```python
from build123d import *

# Parameters (mm, degrees)
F0_R     = 17.65
F0_R_2   = 9.65
F1_DEPTH = 15.2
F2_R     = 0.3
F3_R     = 3.8
F4_DEPTH = 24
F5_R     = 1
F6_R     = 1


with BuildPart() as f1:
    # F0 (on Top) → F1 (new body)
    with BuildSketch(Plane.XY):
        Circle(F0_R)
        Circle(F0_R_2, mode=Mode.SUBTRACT)
    extrude(amount=F1_DEPTH)

    # F2
    f2_edges = [f1.edges().sort_by_distance(p)[0] for p in [
        (-17.65, 0, 15.2),
        (17.65, 0, 7.6),
        (-17.65, 0, 0),
    ]]
    fillet(f2_edges, radius=F2_R)

    # F3 (on Front) → F4 (cut)
    with BuildSketch(Plane.XZ):
        with Locations((0, 7.6)):
            Circle(F3_R)
    extrude(amount=-F4_DEPTH, mode=Mode.SUBTRACT)

    # F5
    f5_edges = [f1.edges().sort_by_distance(p)[0] for p in [
        (-3.8, 17.236081, 7.6),
    ]]
    fillet(f5_edges, radius=F5_R)

    # F6
    f6_edges = [f1.edges().sort_by_distance(p)[0] for p in [
        (-3.8, 8.870316, 7.6),
    ]]
    fillet(f6_edges, radius=F6_R)


solid = f1.part
```
Geometry check sheet. Reference: the model listing, model coordinates, mm. A direction names the side the tool comes from. Give positions to 0.01 mm unless a question says otherwise; leave off trailing zeros. Write each loop counter-clockwise with the first axis right and the second up, starting at its lowest first coordinate (ties: lowest second). Pieces come first, ordered by that corner, then holes. Notation, with made-up numbers: (2, -22) - (12, -22) arc R8 cw to (12, -18) - close; hole circle Ø7 at (39.5, -39). An arc over 180 degrees is marked (long way). Use a Markdown table: item, result.
Q1. Section check B-B, the plane x = 0. Give the number of separate pieces and of enclosed holes in the cut face, then the cut area to 3 significant figures.
Computed:
| item | result |
|---|---|
| separate pieces | 3 |
| enclosed holes | 0 |
| area | 181 mm² |
Q2. Thickness scan on L1, parallel to Z at x = 0, y = 11.5; L2, parallel to X at y = -3, z = 2.25; L3, parallel to Y at x = 0, z = 5.75. Record the ranges inside material, lowest first. Write a range as [from, to].
Computed:
| item | result |
|---|---|
| L1 | z = [0, 3.8], [11.4, 15.2] |
| L2 | x = [-17.39, -9.17], [9.17, 17.39] |
| L3 | y = [-17.65, -9.65] |
Q3. Go/stop test with flat-tipped pins: P1, Ø4, axis at x = 11.5, y = 11.5, coming from the -Z side; P2, Ø7, axis at x = 0, z = 7.6, coming from the +Y side; P3, Ø8, axis at y = 13, z = 13, coming from the +X side. Record where each tip stops, or that it passes through.
Computed:
| item | result |
|---|---|
| P1 | stops at z = 0 |
| P2 | stops at y = -8.99 |
| P3 | stops at x = 15.18 |
Q4. Draft check along X on faces 3 (the face through (7, -7, 0)), 4 (the face through (-3.83, -17.23, 7.5)), 5 (the face through (-2.09, -9.42, 7.49)). Enter one of: pulls with the +X half, pulls with the -X half, needs draft (parallel to the pull), parting line crosses it, or undercut.
Computed:
| item | result |
|---|---|
| face 3 | needs draft |
| face 4 | parting line crosses it |
| face 5 | undercut |
Q5. Section check A-A, the plane y = 0. Enter the section's corners in (x, z), then the cut area to 3 significant figures.
Computed:
| item | result |
|---|---|
| outline | (-17.65, 0.3) arc R0.3 ccw to (-17.35, 0) - (-9.65, 0) - (-9.65, 15.2) - (-17.35, 15.2) arc R0.3 ccw to (-17.65, 14.9) - close; (9.65, 0) - (17.35, 0) arc R0.3 ccw to (17.65, 0.3) - (17.65, 14.9) arc R0.3 ccw to (17.35, 15.2) - (9.65, 15.2) - close |
| area | 243 mm² |
Q6. Section check C-C, the plane z = 1.5. Enter the section's corners in (x, y), then the cut area to 3 significant figures.
Computed:
| item | result |
|---|---|
| outline | circle Ø35.3 at (0, 0); hole circle Ø19.3 at (0, 0) |
| area | 686 mm² |
Q7. Set-up check for faces 1 (the face through (-0.82, 13.02, 3.89)), 2 (the face through (7, -7, 15.2)): record each of +Z, -Z, +X, -X, +Y, -Y from which the full face is reachable in a straight line by a thin tool's end or side.
Computed:
| item | result |
|---|---|
| face 1 | +Y |
| face 2 | +Z, +X, -X, +Y, -Y |
